from build123d import *

# Parameters (mm, degrees)
SKETCH_1_R               = 1.5
SKETCH_1_W               = 15.730611704
SKETCH_1_H               = 11
EXTRUDE_1_DEPTH          = 2
CUT_EXTRUDE_1_DEPTH      = 106.5
CUT_EXTRUDE_1_DEPTH_BACK = 62.743635726
SKETCH_7_R               = 1.2
CUT_EXTRUDE_5_DEPTH      = 15


with BuildPart() as part:
    # Sketch 1 → Extrude 1 (new body)
    with BuildSketch(Plane(origin=(0, 0, 0), x_dir=(1, 0, 0), z_dir=(0, 1, 0))):
        with BuildLine():
            Line((-56.923759365, -23.831956958), (16.382902061, -23.831956958))
            Line((16.382902061, -23.831956958), (-0.836945892, -15.802209985))
            Line((-0.836945892, -15.802209985), (-17.271974735, 0.632818857))
            Line((-17.271974735, 0.632818857), (-55.146365247, 0.632818857))
            ThreePointArc((-55.146365247, 0.632818857), (-50.679018006, -7.808361393), (-51.74094673, -17.29956905))
            ThreePointArc((-51.74094673, -17.29956905), (-53.905020217, -20.904809923), (-56.923759365, -23.831956958))
        make_face()
        with Locations(Location((-43.205666325, -2.789799404, 0), (0, 0, 270))):
            Circle(SKETCH_1_R, mode=Mode.SUBTRACT)
        with Locations(Location((-26.393046621, -2.789799404, 0), (0, 0, 270))):
            Circle(SKETCH_1_R, mode=Mode.SUBTRACT)
        with Locations(Location((-46.193307824, -17.29956905, 0), (0, 0, 270))):
            Circle(SKETCH_1_R, mode=Mode.SUBTRACT)
        with Locations(Location((-22.266173528, -17.29956905, 0), (0, 0, 270))):
            Circle(SKETCH_1_R, mode=Mode.SUBTRACT)
        with Locations((-34.23147938, -13.242579452)):
            Rectangle(SKETCH_1_W, SKETCH_1_H, mode=Mode.SUBTRACT)
    extrude(amount=EXTRUDE_1_DEPTH)

    # Sketch 2 → Cut-Extrude 1 (cut, two sides: drawn at the far end of the back side and taken through both)
    with BuildSketch(Plane(origin=(0, 2, 0), x_dir=(1, 0, 0), z_dir=(0, 1, 0)).offset(-CUT_EXTRUDE_1_DEPTH_BACK)):
        Polygon((16.382902061, -23.831956958), (15.960145161, -23.634822178), (16.059019052, -23.90647596), align=None)
    extrude(amount=CUT_EXTRUDE_1_DEPTH + CUT_EXTRUDE_1_DEPTH_BACK, mode=Mode.SUBTRACT)

    # Sketch 7 → Cut-Extrude 5 (cut)
    with BuildSketch(Plane.XZ):
        with Locations(Location((3.651057562, 21.224691708, 0), (0, 0, 270))):
            Circle(SKETCH_7_R)
    extrude(amount=-CUT_EXTRUDE_5_DEPTH, mode=Mode.SUBTRACT)


solid = part.part
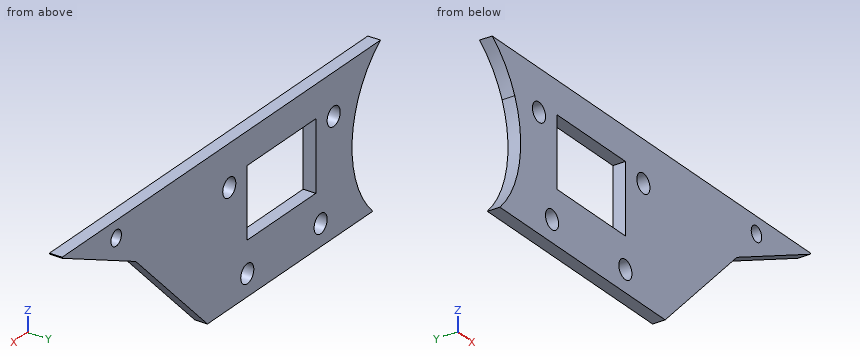
Could you check a few things on this model? Use its own coordinates, in mm. Give positions to 0.01 mm unless a question says otherwise; leave off trailing zeros. Loops run counter-clockwise (first coordinate to the right, second up) from the corner with the lowest first, then second, coordinate; pieces in that order, holes last. Notation, with made-up numbers: M 25.25,-24.5 L 67.25,-24.5 A20 cw 67.25,-13.5 Z; hole C 6,77.25 d9. An arc over 180 degrees is marked long. Answer as a JSON object with one key per item and string values.
Q1. Suppose I cut it at C-C, the plane y = 1.15. List the corners of the cut face in (x, z) for me, plus the area to 3 significant figures.
Values found:
{"outline": "M -56.92,23.83 A16.21 cw -55.15,-0.63 L -17.27,-0.63 L -0.84,15.8 L 15.96,23.63 L 16.03,23.83 Z; hole C -46.19,17.3 d3; hole C -43.21,2.79 d3; hole M -42.1,7.74 L -26.37,7.74 L -26.37,18.74 L -42.1,18.74 Z; hole C -26.39,2.79 d3; hole C -22.27,17.3 d3; hole C 3.65,21.22 d2.4", "area": "983 mm²"}
Q2. If I drill on probe 1 along Z at (x, y) = (-33, 1.75); probe 2 along X at (y, z) = (0.4, 2); probe 3 along X at (y, z) = (0.5, 3.5), over which ranges is the centre line in solid material (lowest first)? Write a range as [from, to].
Values found:
{"probe 1": "z = [-0.63, 7.74], [18.74, 23.83]", "probe 2": "x = [-53.01, -44.48], [-41.93, -27.67], [-25.12, -14.64]", "probe 3": "x = [-52.15, -44.53], [-41.88, -27.71], [-25.07, -13.14]"}
Q3. For P1, Ø0.6, axis at y = 0.5, z = 12, coming from the +X side, with a flat end and sliding along its axis, tell me the tip position at first contact or that it passes through.
Values found:
{"P1": "stops at x = -4.34"}
Q4. Suppose I cut it at B-B, the plane x = -45.5. List the corners of the cut face in (y, z) for me, plus the area to 3 significant figures.
Values found:
{"outline": "M 0,-0.63 L 2,-0.63 L 2,15.97 L 0,15.97 Z; M 0,18.63 L 2,18.63 L 2,23.83 L 0,23.83 Z", "area": "43.6 mm²"}
Q5. Suppose I cut it at A-A, the plane z = 20.75. List the corners of the cut face in (x, y) for me.
Values found:
{"outline": "M -53.78,0 L 2.55,0 L 2.55,2 L -53.78,2 Z; M 4.75,0 L 9.77,0 L 9.77,2 L 4.75,2 Z"}
Q6. Suppose I cut it at D-D, the plane z = 2.5. List the corners of the cut face in (x, y) for me.
Values found:
{"outline": "M -52.7,0 L -44.68,0 L -44.68,2 L -52.7,2 Z; M -41.73,0 L -27.86,0 L -27.86,2 L -41.73,2 Z; M -24.92,0 L -14.14,0 L -14.14,2 L -24.92,2 Z"}
